Verification items for the finished model (mm, model axes). A direction names the side the tool comes from. Coordinates: 2 decimals unless noted, no trailing zeros. Loops run counter-clockwise (first coordinate to the right, second up) from the corner with the lowest first, then second, coordinate; pieces in that order, holes last. Notation, with made-up numbers: (73.25, 48) - (107.25, 48) arc R25 ccw to (107.25, 60) - close; hole circle Ø4 at (-1, 71). An arc over 180 degrees is marked (long way). One line per item, written item: value. Start each with the question number.
(1) Thickness scan on probe 1 along Y at (x, z) = (10, 261) (3 decimals); probe 2 along X at (y, z) = (0, 559); probe 3 along Y at (x, z) = (20, 402). Record the ranges inside material, lowest first. Write a range as [from, to].
(2) Section check B-B (z = 436.5). Record the boundary of the cut face in (x, y).
(3) Section check A-A (x = 25.5). Record the boundary of the cut face in (y, z), plus the area to 3 significant figures.
(4) Gauge pin test, flat ends, axial feed: P1, Ø12, axis at y = 4.5, z = 386.5, coming from the -X side; P2, Ø1, axis at y = -10, z = 208.5, coming from the +X side; P3, Ø5, axis at y = 35, z = 442.5, coming from the +X side. Record the tip position at first contact, or that the pin passes through.
(5) Set-up check for faces 1 (the face through (27.317, 42.385, 319.674)), 2 (the face through (23, 50, 320)): record each of +Z, -Z, +X, -X, +Y, -Y from which the full face is reachable in a straight line by a thin tool's end or side.
(6) Section check C-C (y = 21.5). Record the boundary of the cut face in (x, z).
Autodesk Inventor part; units mm, degrees
ref_plane "Начальная плоскость" through (0, 0, -23) normal (0, 0, 1) x (1, 0, 0)
ref_plane "Конечная плоскость" through (0, 0, 672) normal (0, 0, 1) x (1, 0, 0)
ref_plane "РабПлоскость8" through (46, 0, 672) normal (-0.7071, 0, 0.7071) x (0.7071, 0, 0.7071)
ref_plane "Начальная плоскость" through (0, 0, -23) normal (0, 0, 1) x (1, 0, 0)
ref_plane "Конечная плоскость" through (0, 0, 672) normal (0, 0, 1) x (1, 0, 0)
sketch "Эскиз" plane through (0, 0, 0) normal (0, 0, 1) x (1, 0, 0)
  line L0 (46, -50) -> (0, -50)
  line L1 (46, -50) -> (46, -46.6496)
  line L2 (43.2392, -43.6591) -> (10.9418, -41.0753)
  line L3 (4.5, -34.0976) -> (4.5, 34.0976)
  line L4 (43.2392, 43.6591) -> (10.9418, 41.0753)
  line L5 (46, 46.6496) -> (46, 50)
  line L6 (0, 50) -> (46, 50)
  line L7 (0, -50) -> (0, 50)
  arc A0 (4.5, -34.0976) -> (10.9418, -41.0753) centre (11.5, -34.0976) ccw
  arc A1 (10.9418, 41.0753) -> (4.5, 34.0976) centre (11.5, 34.0976) ccw
  arc A2 (46, -46.6496) -> (43.2392, -43.6591) centre (43, -46.6496) ccw
  arc A3 (43.2392, 43.6591) -> (46, 46.6496) centre (43, 46.6496) ccw
  line L8 (0, 70) -> (0, -70) construction
  line L9 (-9.3169, 0) -> (55.9016, 0) construction
  point P0 (46, -43.88)
  point P1 (4.5, -40.56)
  point P2 (4.5, 40.56)
  point P3 (46, 43.88)
  dimension "d3" = 46
  dimension "d5" = 4.5
  dimension "d7" = 100
  dimension "d9" = 9.44
  dimension "d11" = 9.44
  dimension "d13" = 6.12
  dimension "d15" = 6.12
  dimension "d22" = 7
  dimension "d23" = 3
  dimension "d24" = 50
  dimension "d25" = 0
extrude "Тело" add sketch "Эскиз" along normal up to surface (695 mm away) from surface at -23
sketch "Sketch3" plane through (0, 0, 0) normal (0, 0, 1) x (1, 0, 0)
  line L0 (0, 0) -> (10, 0)
ref_plane "Work Plane7" through (0, 0, 0) normal (0, -1, 0) x (1, 0, 0)
sketch "Sketch4" plane through (0, 0, 0) normal (0, -1, 0) x (1, 0, 0)
  line L0 (-2, -23) -> (12, -23)
  line L1 (-2, 672) -> (12, 672)
  dimension "d29" = 695
ref_plane "РабПлоскость8" through (46, 0, 672) normal (-0.7071, 0, 0.7071) x (0.7071, 0, 0.7071)
split "Разделение1" plane through (46, 0, 672) removes the side toward (-0.7071, 0, 0.7071)
ref_plane "РабПлоскость9" through (46, 0, -23) normal (-0.7071, 0, -0.7071) x (-0.7071, 0, 0.7071)
split "Разделение2" plane through (46, 0, -23) removes the side toward (-0.7071, 0, -0.7071)
equation "\"d3\" = b"
equation "\"d7\" = ParH"
equation "\"d22\" = R"
equation "\"d23\" = R1"
equation "\"d24\" = 0.5 * d7"
equation "\"d16\" = G_L"
equation "\"R1\" = 3"
equation "\"R\" = 7"
equation "\"t1\" = 4.5"
equation "\"t2\" = 7.6"
equation "\"ParH\" = 100"
equation "\"b\" = 46"
equation "\"msp_x1\" = 0.04 * b"
equation "\"msp_x2\" = -0.08 * t1 + 0.04 * b"
equation "\"G_L\" = d29"
equation "\"ex\" = 0"
equation "\"G_OFFSET_START\" = 23"
equation "\"G_OFFSET_END\" = 23"
equation "\"d26\" = -G_OFFSET_START"
equation "\"d27\" = G_OFFSET_END + B_L"
equation "\"B_L\" = 649"
properties part number "Швеллер 10U-695 ГОСТ 8240-97" material "Сталь, мягкая"
Responses:
1. probe 1: y = [-50, -40.935], [40.935, 50]
1. probe 2: x = [0, 4.5]
1. probe 3: y = [-50, -41.8], [41.8, 50]
2. outline: (0, -50) - (46, -50) - (46, -46.65) arc R3 ccw to (43.24, -43.66) - (10.94, -41.08) arc R7 cw to (4.5, -34.1) - (4.5, 34.1) arc R7 cw to (10.94, 41.08) - (43.24, 43.66) arc R3 ccw to (46, 46.65) - (46, 50) - (0, 50) - close
3. outline: (-50, -2.5) - (-42.24, -2.5) - (-42.24, 651.5) - (-50, 651.5) - close; (42.24, -2.5) - (50, -2.5) - (50, 651.5) - (42.24, 651.5) - close
3. area: 10,200 mm²
4. P1: stops at x = 0
4. P2: stops at x = 4.5
4. P3: stops at x = 5.38
5. face 1: +Z, -Z, +X
5. face 2: +Z, -Z, +X, -X, +Y
6. outline: (0, 23) - (4.5, 18.5) - (4.5, 630.5) - (0, 626) - close
